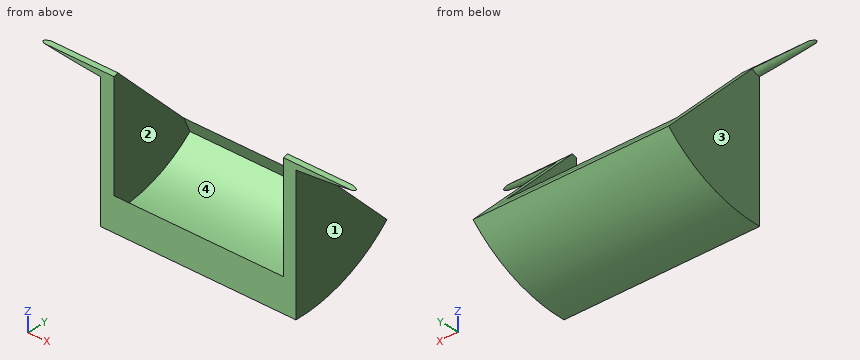
from build123d import *

# Parameters (mm, degrees)
REVOLVE1_ANGLE            = 45
CUT_REVOLVE_THIN3_START   = -65.672494398
CUT_REVOLVE_THIN3_DEPTH   = 132.08
CUT_REVOLVE_THIN3_START_2 = 59.247024
CUT_REVOLVE_THIN3_2_DEPTH = 7.160481602
EXTRUDE_THIN1_DEPTH       = 132.08
BOSS_EXTRUDE1_START       = 132.08
BOSS_EXTRUDE1_DEPTH       = 132.08
SKETCH12_R                = 990.316340453
CUT_EXTRUDE1_DEPTH        = 132.08
SKETCH14_W                = 3.086900102
SKETCH14_H                = 1.742063617
CUT_EXTRUDE5_DEPTH        = 2.54
SKETCH16_R                = 990.316340453
CUT_EXTRUDE6_DEPTH        = 351.028


# Read off the part's stored shape, not the designer's step: Cut-Revolve-Thin3
with BuildPart() as part:
    # Sketch1 → Revolve1 (revolve)
    with BuildSketch(Plane(origin=(0, 0, 0), x_dir=(1, 0, 0), z_dir=(0, 1, 0))):
        with BuildLine():
            Line((76.2, 994.033632479), (76.2, 1095.633632479))
            Line((76.2, 1095.633632479), (-76.2, 1095.633632479))
            Line((-76.2, 1095.633632479), (-76.2, 994.033632479))
            ThreePointArc((-76.2, 994.033632479), (-114.384675321, 990.366320384), (-152.4, 985.232735195))
            Line((-152.4, 985.232735195), (-102.9796946, 985.232735195))
            ThreePointArc((-102.9796946, 985.232735195), (0, 990.6), (102.9796946, 985.232735195))
            Line((102.9796946, 985.232735195), (152.4, 985.232735195))
            ThreePointArc((152.4, 985.232735195), (114.384675321, 990.366320384), (76.2, 994.033632479))
        make_face()
    revolve(axis=Axis((-102.9796946, 0, -985.232735195), (1, 0, 0)), revolution_arc=REVOLVE1_ANGLE)

    # Cut-Revolve-Thin3 outline → Cut-Revolve-Thin3 (cut)
    with BuildSketch(Plane.YZ.offset(CUT_REVOLVE_THIN3_START)):
        with BuildLine():
            ThreePointArc((0, -1082.04), (37.046536374, -1074.670985747), (68.453073412, -1053.685808607))
            Line((68.453073412, -1053.685808607), (2.371248163, -987.603983358))
            ThreePointArc((2.371248163, -987.603983358), (1.283310258, -988.330920225), (0, -988.586186506))
            Line((0, -988.586186506), (0, -1082.04))
        make_face()
    extrude(amount=CUT_REVOLVE_THIN3_DEPTH, mode=Mode.SUBTRACT)

    # Cut-Revolve-Thin3 2 outline → Cut-Revolve-Thin3 2 (cut)
    with BuildSketch(Plane.YZ.offset(CUT_REVOLVE_THIN3_START_2)):
        with BuildLine():
            ThreePointArc((0, -988.586186506), (1.283310258, -988.330920225), (2.371248163, -987.603983358))
            Line((2.371248163, -987.603983358), (2.337863382, -987.570598578))
            ThreePointArc((2.337863382, -987.570598578), (1.265242545, -988.287300908), (0, -988.538973298))
            Line((0, -988.538973298), (0, -988.586186506))
        make_face()
    extrude(amount=CUT_REVOLVE_THIN3_2_DEPTH, mode=Mode.SUBTRACT)

    # Sketch5 → Extrude-Thin1 (add)
    with BuildSketch(Plane(origin=(-65.672494398, 0, 0), x_dir=(0, 0, -1), z_dir=(1, 0, 0))):
        Polygon((1082.04, 0), (1070.380989237, 0), (1081.891098133, 5.367251924), (1082.964548518, 3.065230145), (1081.838188837, 2.54), (1082.04, 2.54), align=None)
    extrude(amount=EXTRUDE_THIN1_DEPTH)

    # Sketch11 → Boss-Extrude1 (add)
    with BuildSketch(Plane.ZY.offset(-66.407505602).offset(BOSS_EXTRUDE1_START)):
        with BuildLine():
            Line((-1053.685808607, 68.453073412), (-1045.195024303, 59.962289107))
            Line((-1045.195024303, 59.962289107), (-1056.738187334, 65.258078683))
            ThreePointArc((-1056.738187334, 65.258078683), (-1055.230229553, 66.872993821), (-1053.685808607, 68.453073412))
        make_face()
    extrude(amount=-BOSS_EXTRUDE1_DEPTH)

    # Sketch12 → Cut-Extrude1 (cut)
    with BuildSketch(Plane(origin=(-65.672494398, 0, 0), x_dir=(0, 0, -1), z_dir=(1, 0, 0))):
        with Locations((48.724048718, -308.713234064)):
            Circle(SKETCH12_R)
    extrude(amount=-CUT_EXTRUDE1_DEPTH, mode=Mode.SUBTRACT)


with BuildPart() as cut_extrude1_piece_1:
    # of the separate pieces the step leaves, piece 1, a body of its own (cut_extrude1_pieces)
    add(part.part.solids().sort_by_distance((152.4, 0, -985.232735195))[0])

    # Sketch16 → Cut-Extrude6 (cut)
    with BuildSketch(Plane(origin=(-65.672494398, 0, 0), x_dir=(0, 0, -1), z_dir=(1, 0, 0))):
        with Locations((48.724048718, -308.713234064)):
            Circle(SKETCH16_R)
    extrude(amount=CUT_EXTRUDE6_DEPTH, mode=Mode.SUBTRACT)


with BuildPart() as cut_extrude1_piece_2:
    # of the separate pieces the step leaves, piece 2, a body of its own (cut_extrude1_pieces)
    add(part.part.solids().sort_by_distance((-65.672494398, 0, -988.586186506))[0])

    # Sketch14 → Cut-Extrude5 (cut)
    with BuildSketch(Plane.XZ):
        with Locations((-64.129044347, -987.715154698)):
            Rectangle(SKETCH14_W, SKETCH14_H)
    extrude(amount=-CUT_EXTRUDE5_DEPTH, mode=Mode.SUBTRACT)


solid = cut_extrude1_piece_1.part
For this review, take the finished solid that the model builds, in its own axes (mm). Face numbers are marked on the shaded views. Give positions to 0.01 mm unless a question says otherwise; leave off trailing zeros. Order: outer loops, then holes, each group sorted by start corner. A loop starts at its lowest first (then second) coordinate and runs counter-clockwise, first axis right, second up. Notation, with made-up numbers: M 86.25,-9.75 L 140.25,-9.75 A22 cw 140.25,21.25 Z; hole C 73,-27 d7. An arc over 180 degrees is marked long. Answer in a Markdown table with one row per item. Add a question column.
(1) Consider section A-A on z = -1036.5. State the section outline as (x, y) points.
(2) Mouldability with a two-part tool opening along X and no side actions: class the marked faces 1, 2, 3 and 4 as +X half, -X half, draft (parallel to the pull), parting line (faces both ways), or undercut.
(3) Wall thickness on probe 1 along X at (y, z) = (27, -1038.5); probe 2 along X at (y, z) = (29, -1081); probe 3 along Y at (x, z) = (6, -1073): over which ranges is each line inside the solid? List them lowest first. Write a range as [from, to].
(4) Consider section C-C on y = 30. State the section outline as (x, z) points, and give its area (3 significant figures).
(5) For pin 1 (1.5 mm diameter, centred on y = 41.5, z = -1041.5, fed in from -X); pin 2 (10 mm diameter, centred on y = 12.5, z = -1053, fed in from +X); pin 3 (6 mm diameter, centred on x = 29.5, y = 18.5, fed in from +Z), all flat-tipped, find the tip position at first contact; note any pin that passes through.
(6) Consider section D-D on z = -1077.5. State the section outline as (x, y) points.
Evaluation:
| question | item | result |
|---|---|---|
| 1 | outline | M -76.2,0 L -65.67,0 L -65.67,51.27 L -76.2,51.27 Z; M 66.41,0 L 76.2,0 L 76.2,51.27 L 66.41,51.27 Z |
| 2 | face 1 | +X half |
| 2 | face 2 | undercut |
| 2 | face 3 | -X half |
| 2 | face 4 | undercut |
| 3 | probe 1 | x = [-76.2, -65.67], [66.41, 76.2] |
| 3 | probe 2 | x = [-76.2, 76.2] |
| 3 | probe 3 | y = [0, 1.22], [40.85, 66.97] |
| 4 | outline | M -76.2,-1091.48 L 76.2,-1091.48 L 76.2,-1015.23 L 66.41,-1015.23 L 66.41,-1077.27 L -65.67,-1077.27 L -65.67,-1015.23 L -76.2,-1015.23 Z |
| 4 | area | 3,430 mm^2 |
| 5 | pin 1 | stops at x = -76.2 |
| 5 | pin 2 | stops at x = 76.2 |
| 5 | pin 3 | stops at z = -1079.62 |
| 6 | outline | M -76.2,0 L 76.2,0 L 76.2,60.62 L -76.2,60.62 Z; hole M -65.67,3.32 L 66.41,3.32 L 66.41,29.3 L -65.67,29.3 Z |
